Geometry: see drawing. Coordinates: mm, zero at the bounding-box minimum. A direction names the side the tool comes from. Coordinates: 2 decimals unless noted, no trailing zeros. Write each loop counter-clockwise with the first axis right and the second up, starting at its lowest first coordinate (ties: lowest second). Pieces come first, ordered by that corner, then holes.
1) Line query: L1, parallel to X at y = 18, z = 18.5; L2, parallel to Z at x = 32, y = 35. Output: solid intervals per line, ascending.
2) Section query D-D (x = 85.5). Output: boundary loops of the cut face in (y, z).
3) Section query A-A (z = 37.5). Output: boundary loops of the cut face in (x, y), then the cut area to 3 significant figures.
4) Pin query (flat end, axial travel): pin 1 Ø3 at (y, z) = (20, 43) entering from -X. Return the tip coordinate at first contact, or that it passes through.
5) Section query C-C (y = 9.5). Output: boundary loops of the cut face in (x, z), then the cut area to 3 significant figures.
6) Set-up query: the marked faces 1 and 2. Return all of +Z, -Z, +X, -X, +Y, -Y with unobstructed straight access to the full face (end or side cutting, diameter ignored); none if empty.
7) Section query B-B (x = 72). Output: boundary loops of the cut face in (y, z).
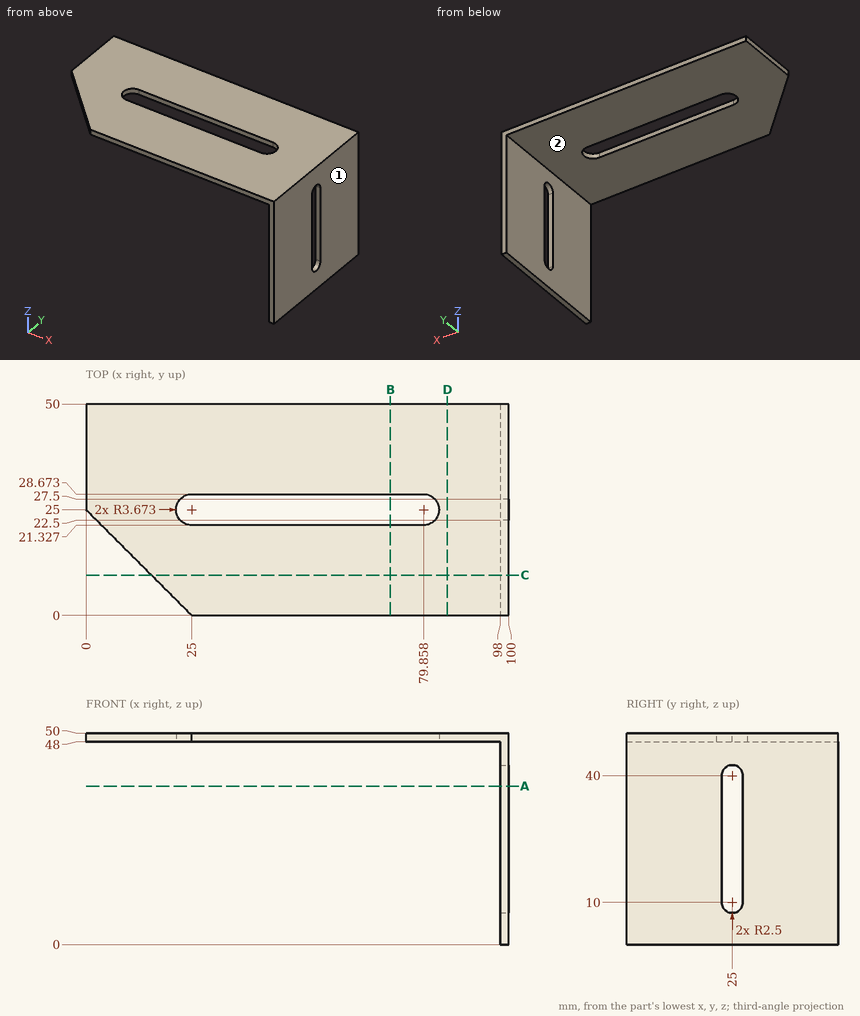
Answer:
1. L1: x = 98 to 100
1. L2: z = 48 to 50
2. outline: (0, 48) - (50, 48) - (50, 50) - (0, 50) - close
3. outline: (98, 0) - (100, 0) - (100, 22.5) - (98, 22.5) - close; (98, 27.5) - (100, 27.5) - (100, 50) - (98, 50) - close
3. area: 90.0 mm2
4. pin 1: stops at x = 98
5. outline: (15.5, 48) - (98, 48) - (98, 0) - (100, 0) - (100, 50) - (15.5, 50) - close
5. area: 265 mm2
6. face 1: +Z, -Z, +X, +Y, -Y
6. face 2: -Z, -X, +Y, -Y
7. outline: (0, 48) - (21.33, 48) - (21.33, 50) - (0, 50) - close; (28.67, 48) - (50, 48) - (50, 50) - (28.67, 50) - close
